Here's how the part is built. I have some questions about the finished solid (model axes, mm). Coordinates: 2 decimals unless noted, no trailing zeros. Write each loop counter-clockwise with the first axis right and the second up, starting at its lowest first coordinate (ties: lowest second). Pieces come first, ordered by that corner, then holes. Notation, with made-up numbers: (76, 45) - (118, 45) arc R6 cw to (118, 51) - close; hole circle Ø8 at (-17.75, 87.25). An arc over 180 degrees is marked (long way). Answer in a Markdown table with one row per item. Add a question column.
Item 1: We'd pull the mould along Z, two halves only. Please class faces 1 (the face through (2, 0, 8)), 2 (the face through (2.472, -2.83, 3.087)), 3 (the face through (5, 2, -5)): +Z half, -Z half, draft (parallel to the pull), parting line (faces both ways), or undercut.
Item 2: If I drill on probe 1 along Z at (x, y) = (2.2, 0); probe 2 along Y at (x, z) = (4.15, -1.75); probe 3 along Y at (x, z) = (3.55, -1.5), over which ranges is the centre line in solid material (lowest first)? Write a range as from..to.
Item 3: Imagine slicing it at A-A (y = 0). Please give me the cut outline in (x, z), plus the area to 3 significant figures.
Item 4: Imagine slicing it at B-B (x = 2.9). Please give me the cut outline in (y, z), plus the area to 3 significant figures.
Item 5: I'm going to push flat-ended pins straight in: pin 1 (1 mm diameter, centred on x = 2, z = -5, fed in from +Y); pin 2 (2 mm diameter, centred on x = 2, z = -1.5, fed in from -Y). Where does each tip first touch, or does it pass through?
Autodesk Inventor part; units mm, degrees
ref_plane "Work Plane1" through (-20.0362, 0, 0) normal (0, -0.866, -0.5) x (1, 0, 0)
ref_plane "YZ Plane" through (0, 0, 0) normal (1, 0, 0) x (0, 1, 0)
ref_plane "XZ Plane" through (0, 0, 0) normal (0, 1, 0) x (-1, 0, 0)
sketch "Sketch1" plane through (0, 0, 0) normal (1, 0, 0) x (0, 1, 0)
  line L0 (-9.2376, 0) -> (-4.6188, 8)
  line L1 (-4.6188, 8) -> (4.6188, 8)
  line L2 (4.6188, 8) -> (9.2376, 0)
  line L3 (9.2376, 0) -> (4.6188, -8)
  line L4 (4.6188, -8) -> (-4.6188, -8)
  line L5 (-4.6188, -8) -> (-9.2376, 0)
  point P0 (0, 0)
  point P1 (0, 0)
  dimension "d0" = 18.4752
extrude "Body" add sketch "Sketch1" along normal blind 5
sketch "Sketch2" plane through (0, 0, 0) normal (0, 0, 1) x (1, 0, 0)
  line L0 (0, 4.6188) -> (0, 9.2376)
  line L1 (0, 9.2376) -> (5, 9.2376)
  line L2 (5, 4.6188) -> (5, 9.2376)
  line L3 (-1, 0) -> (6, 0)
  line L4 (1.1187, 9.2376) -> (0, 7.3)
  line L5 (3.8813, 9.2376) -> (5, 7.3)
  dimension "d3" = 30
  dimension "d4" = 30
  dimension "d5" = 14.6
  dimension "d6" = 14.6
revolve "Chamfer1" cut sketch "Sketch2" angle 360 about axis through (-10, 0, 0) along (1, 0, 0)
sketch "Sketch3" plane through (5, 0, 0) normal (1, 0, 0) x (0, 0, -1)
  arc A0 (-0.625, -1.0825) -> (0.625, -1.0825) centre (0, 0) ccw
hole "Thread" at (5, 0, 0) direction (-1, 0, 0) diameter 8.376 end through all
chamfer "Chamfer2" distance 0.8119 angle 30 1 edges at (5, 0, 4.188) measured on face at (5, 6.1818, -0.7506)
chamfer "Chamfer3" distance 0.8119 angle 30 1 edges at (0, 0, 4.188) measured on face at (0, 6.1818, -0.7506)
ref_plane "Work Plane1" through (-20.0362, 0, 0) normal (0, -0.866, -0.5) x (1, 0, 0)
equation "\"d0\" = 1.1547 * SW"
equation "\"d1\" = KOH"
equation "\"d3\" = ANG1"
equation "\"d4\" = ANG2"
equation "\"d5\" = SW0"
equation "\"d6\" = SW01"
equation "\"d8\" = -0.5 * GD1 + 0.5 * NND"
equation "\"d40\" = -0.5 * GD1 + 0.5 * NND"
equation "\"d10\" = -0.5 * GD1 + 0.5 * NND"
equation "\"d41\" = -0.5 * GD1 + 0.5 * NND"
equation "\"ANG1\" = 30deg"
equation "\"ANG2\" = 30deg"
equation "\"KOH\" = 5"
equation "\"SW\" = 16"
equation "\"SW0\" = 14.6"
equation "\"SW01\" = SW0"
equation "\"GUL\" = 0.541266 * PTC"
equation "\"TOA\" = 30deg"
equation "\"PTC\" = 1.5"
equation "\"E0\" = 1.155 * SW"
equation "\"GAL\" = 0.541266 * PTC"
properties part number "ISO 4035 - M10" material "Stainless Steel, 440C"
Here are the results:
| question | item | result |
|---|---|---|
| 1 | face 1 | +Z half |
| 1 | face 2 | undercut |
| 1 | face 3 | draft |
| 2 | probe 1 | z = -8..-4.19, 4.19..8 |
| 2 | probe 2 | y = -8.23..-3.8, 3.8..8.23 |
| 2 | probe 3 | y = -8.37..-3.91, 3.91..8.37 |
| 3 | outline | (0, -7.3) - (0.4, -8) - (4.6, -8) - (5, -7.3) - (5, -5) - (4.53, -4.19) - (0.47, -4.19) - (0, -5) - close; (0, 5) - (0.47, 4.19) - (4.53, 4.19) - (5, 5) - (5, 7.3) - (4.6, 8) - (0.4, 8) - (0, 7.3) - close |
| 3 | area | 36.8 mm2 |
| 4 | outline | (-9.24, 0) - (-4.62, -8) - (4.62, -8) - (9.24, 0) - (4.62, 8) - (-4.62, 8) - close; hole circle Ø8.38 at (0, 0) |
| 4 | area | 167 mm2 |
| 5 | pin 1 | stops at y = 6.64 |
| 5 | pin 2 | stops at y = -8.95 |
